Model file for the job. Use its own axes, mm. A direction names the side the tool comes from. Round coordinates to 2 decimals unless told otherwise and drop trailing zeros. Loops run counter-clockwise (first coordinate to the right, second up) from the corner with the lowest first, then second, coordinate; pieces in that order, holes last. Notation, with made-up numbers: (-7, -23.5) - (36, -23.5) arc R29 ccw to (36, -0.5) - close; hole circle Ø6 at (83, 63). An arc over 180 degrees is marked (long way). Use one line per item in the form item = value.
from build123d import *

# Parameters (mm, degrees)
F0_W     = 46.244312
F0_H     = 39.637983
F1_DEPTH = 5
F2_W     = 60
F2_H     = 40
F3_DEPTH = 30
F5_DEPTH = 25
F8_DEPTH = 36


with BuildPart() as f1:
    # F0 (on Front) → F1 (new body)
    with BuildSketch(Plane.XZ):
        with Locations((-23.122156, 19.818991)):
            Rectangle(F0_W, F0_H)
    extrude(amount=F1_DEPTH)

    # F2 (on face) → F3 (join)
    with BuildSketch(Plane.XZ.offset(5)):
        with Locations((-30, -0.181009)):
            Rectangle(F2_W, F2_H)
    extrude(amount=-F3_DEPTH)

    # F4 (on face) → F5 (join)
    with BuildSketch(Plane(origin=(0, 25, 0), x_dir=(-1, 0, 0), z_dir=(0, 1, 0))):
        with BuildLine():
            ThreePointArc((79.248183, -0.181009), (73.610521, 13.429512), (60, 19.067175))
            Line((60, 19.067175), (60, -19.429192))
            ThreePointArc((60, -19.429192), (73.610521, -13.79153), (79.248183, -0.181009))
        make_face()
    extrude(amount=-F5_DEPTH)

    # F6: F1 across plane


with BuildPart() as f1_1:
    add(f1.part)
    add(f1.part.mirror(Plane.YZ))

    # F7 (on face) → F8 (join)
    with BuildSketch(Plane(origin=(0, 25, 0), x_dir=(-1, 0, 0), z_dir=(0, 1, 0))):
        Polygon((11.674208, -13.803926), (53.077161, 0), (18.913604, 10.272454), align=None)
    extrude(amount=F8_DEPTH)


solid = f1_1.part
1. Flat gauge pins, fed straight in: pin 1 (6 mm diameter, centred on y = 30, z = 0, fed in from +X); pin 2 (21 mm diameter, centred on x = 67, z = -9, fed in from -Y); pin 3 (5.5 mm diameter, centred on y = -1.5, z = 34, fed in from -X); pin 4 (6 mm diameter, centred on x = -66, z = -4.5, fed in from -Y). Where does each tip first touch, or does it go through?
Geometry check:
pin_1 = -14.92
pin_2 = -5
pin_3 = -46.24
pin_4 = 0
2. Cut at C-C, the plane z = 5.5. Give the cut face in (x, y).
Geometry check:
outline = (-78.39, 0) - (-60, 0) - (-60, -5) - (60, -5) - (60, 0) - (78.39, 0) - (78.39, 25) - (-17.48, 25) - (-17.48, 61) - (-34.79, 61) - (-34.79, 25) - (-78.39, 25) - close
3. Tool access for faces 1 (the flat face through (46.244, -2, 30)), 2 (the flat face through (67, 0, 0)), 3 (the flat face through (-67, 0, 0)), 4 (the flat face through (-46.244, -2, 30)), 5 (the flat face through (1, 0, 30)): list every direction of +Z, -Z, +X, -X, +Y, -Y with a clear straight run to the whole face (end or side of a thin tool).
Geometry check:
face_1 = +Z, +X, +Y, -Y
face_2 = +Z, -Z, +X, -Y
face_3 = +Z, -Z, -X, -Y
face_4 = +Z, -X, +Y, -Y
face_5 = +Z, +X, -X, +Y
4. Cut at B-B, the plane x = 33. Give the cut face in (y, z).
Geometry check:
outline = (-5, -20.18) - (25, -20.18) - (25, 19.82) - (0, 19.82) - (0, 39.64) - (-5, 39.64) - close
5. Cut at A-A, the plane y = 18.5. Give the cut face in (x, z).
Geometry check:
outline = (-79.25, -0.18) arc R19.25 ccw to (-60, -19.43) - (-60, -20.18) - (60, -20.18) - (60, -19.43) arc R19.25 ccw to (79.25, -0.18) arc R19.25 ccw to (60, 19.07) - (60, 19.82) - (-60, 19.82) - (-60, 19.07) arc R19.25 ccw to start
6. Cut at D-D, the plane z = -10. Give the cut face in (x, y), plus the area to 3 significant figures.
Geometry check:
outline = (-76.56, 0) - (-60, 0) - (-60, -5) - (60, -5) - (60, 0) - (76.56, 0) - (76.56, 25) - (-12.82, 25) - (-12.82, 61) - (-23.08, 61) - (-23.08, 25) - (-76.56, 25) - close
area = 4,800 mm^2
7. Wall check: probe 1 along Y at (x, z) = (-39.5, -10); probe 2 along Y at (x, z) = (-68, 16.5); probe 3 along Z at (x, y) = (2, 19.5). Give the ranges that are in metal, low to high.
Geometry check:
probe_1 = -5 to 25
probe_2 = 0 to 25
probe_3 = -20.18 to 19.82
